Model file for the job. Use its own axes, mm. A direction names the side the tool comes from. Round coordinates to 2 decimals unless told otherwise and drop trailing zeros. Order: outer loops, then holes, each group sorted by start corner. A loop starts at its lowest first (then second) coordinate and runs counter-clockwise, first axis right, second up. Notation, with made-up numbers: (11.25, 28) -> (18.25, 28) arc R26 ccw to (18.25, 60) -> close; hole circle Ø11 at (84, -19). An arc over 180 degrees is marked (long way). Put each result on its own line as item: value. Start each with the question number.
Q1. Cut at C-C, the plane z = 5. List the corners of the cut face in (x, y).
Q2. 3-axis set-ups, long thin cutter, end or side, ignore diameter. For faces 4 (the face through (8, 0.6, 6)), 5 (the face through (5.356, 2.276, 5.062)), 6 (the face through (0, -4, 5)): which of +Z, -Z, +X, -X, +Y, -Y reach the whole face in a straight line?
Q3. Cut at D-D, the plane x = 6.5. State how many separate pieces and enclosed holes the cut face has, and give its area (3 significant figures).
Q4. Cut at B-B, the plane y = 0. List the corners of the cut face in (x, z).
Q5. Pull direction Z, two halves, no side cores. Call faces 1 (the face through (0.08, 4.13, 0.62)), 2 (the face through (3.257, 6.083, 4.886)), 3 (the face through (0, 4, 5)): released by +Z, released by -Z, zero draft, split by the parting line, or undercut.
Q6. Cut at A-A, the plane x = 0. List the corners of the cut face in (y, z), and give its area (3 significant figures).
Q7. Flat gauge pins, fed straight in: P1, Ø1, axis at x = -7, z = 1.5, coming from the -Y side; P2, Ø3, axis at x = 6.5, z = 3.5, coming from the +Y side; P3, Ø1, axis at x = -5.5, z = 2.5, coming from the -Y side. Where does each tip first touch, or does it go through?
Q8. Probe L1, parallel to Y at x = 0, z = 2.5; L2, parallel to X at y = 1.5, z = 4.5; L3, parallel to Z at x = 7.5, y = -3. List the from-to ranges inside material, lowest first.
from build123d import *

# Parameters (mm, degrees)
SKICA1_R                 = 10
SKICA1_R_2               = 4
P_IDAT_VYSUNUT_M1_DEPTH  = 10
ODEBRAT_VYSUNUT_M1_DEPTH = 10
SKICA3_R                 = 1.375
ODEBRAT_VYSUNUT_M2_DEPTH = 10
SKICA4_R                 = 1.4
ODEBRAT_VYSUNUT_M3_DEPTH = 10
SKICA5_R                 = 3.5
ODEBRAT_VYSUNUT_M4_DEPTH = 10
ZAOBLIT1_R               = 1
ZKOSEN_2_SIZE            = 0.75


with BuildPart() as part:
    # Skica1 → Přidat vysunutím1 (new body)
    with BuildSketch(Plane.XY):
        Circle(SKICA1_R)
        Circle(SKICA1_R_2, mode=Mode.SUBTRACT)
    extrude(amount=P_IDAT_VYSUNUT_M1_DEPTH)

    # Skica2 → Odebrat vysunutím1 (cut)
    with BuildSketch(Plane.XY.offset(10)):
        with BuildLine():
            Line((-7.225129757, 0.6), (12.11079591, 0.6))
            Line((12.11079591, 0.6), (12.11079591, -0.6))
            Line((12.11079591, -0.6), (-7.225129757, -0.6))
            ThreePointArc((-7.225129757, -0.6), (-7.25, 0), (-7.225129757, 0.6))
        make_face()
    extrude(amount=-ODEBRAT_VYSUNUT_M1_DEPTH, mode=Mode.SUBTRACT)

    # Skica3 → Odebrat vysunutím2 (cut)
    with BuildSketch(Plane(origin=(0, -0.6, 0), x_dir=(1, 0, 0), z_dir=(0, 1, 0))):
        with Locations(Location((6.754743987, -5, 0), (0, 0, 180))):
            Circle(SKICA3_R)
    extrude(amount=-ODEBRAT_VYSUNUT_M2_DEPTH, mode=Mode.SUBTRACT)

    # Skica4 → Odebrat vysunutím3 (cut)
    with BuildSketch(Plane.XZ.offset(-0.6)):
        with Locations((6.754743987, 5)):
            Circle(SKICA4_R)
    extrude(amount=-ODEBRAT_VYSUNUT_M3_DEPTH, mode=Mode.SUBTRACT)

    # Skica5 → Odebrat vysunutím4 (cut)
    with BuildSketch(Plane(origin=(0, 4, 0), x_dir=(1, 0, 0), z_dir=(0, 1, 0))):
        with Locations((6.754743987, -5)):
            Circle(SKICA5_R)
    extrude(amount=ODEBRAT_VYSUNUT_M4_DEPTH, mode=Mode.SUBTRACT)

    # Zaoblit1
    zaoblit1_edges = [part.edges().sort_by_distance(p)[0] for p in [
        (-10, 0, 0),
        (-10, 0, 10),
    ]]
    fillet(zaoblit1_edges, radius=ZAOBLIT1_R)

    # Zkosení2
    zkosen_2_edges = [part.edges().sort_by_distance(p)[0] for p in [
        (0, -4, 10),
        (0, -4, 0),
        (0, 4, 0),
        (0, 4, 10),
    ]]
    chamfer(zkosen_2_edges, length=ZKOSEN_2_SIZE)


solid = part.part
Ans:
1. outline: (-7.23, -0.6) arc R7.25 cw to (-7.23, 0.6) -> (-3.95, 0.6) arc R4 cw to (3.95, 0.6) -> (5.35, 0.6) -> (5.35, 4) -> (3.25, 4) -> (3.25, 9.46) arc R10 ccw (long way) to (5.38, -8.43) -> (5.38, -0.6) -> (3.95, -0.6) arc R4 cw to (-3.95, -0.6) -> close; (8.13, -5.82) arc R10 ccw to (9.98, -0.6) -> (8.13, -0.6) -> close; (8.15, 0.6) -> (9.98, 0.6) arc R10 ccw to (9.17, 4) -> (8.15, 4) -> close
2. face 4: +Z, -Z, +X
2. face 5: +Y
2. face 6: +Z, -Z
3. separate pieces: 4
3. enclosed holes: 0
3. area: 85.4 mm^2
4. outline: (-10, 1) arc R1 ccw to (-9, 0) -> (-7.25, 0) -> (-7.25, 10) -> (-9, 10) arc R1 ccw to (-10, 9) -> close
5. face 1: released by -Z
5. face 2: undercut
5. face 3: zero draft
6. outline: (-10, 1) arc R1 ccw to (-9, 0) -> (-4.75, 0) -> (-4, 0.75) -> (-4, 9.25) -> (-4.75, 10) -> (-9, 10) arc R1 ccw to (-10, 9) -> close; (4, 0.75) -> (4.75, 0) -> (9, 0) arc R1 ccw to (10, 1) -> (10, 9) arc R1 ccw to (9, 10) -> (4.75, 10) -> (4, 9.25) -> close
6. area: 118 mm^2
7. P1: stops at y = -7.6
7. P2: stops at y = 4
7. P3: stops at y = -8.66
8. L1: y = -10 to -4, 4 to 10
8. L2: x = -9.89 to -3.71, 3.71 to 5.45, 8.06 to 9.89
8. L3: z = 0 to 3.84, 6.16 to 10
